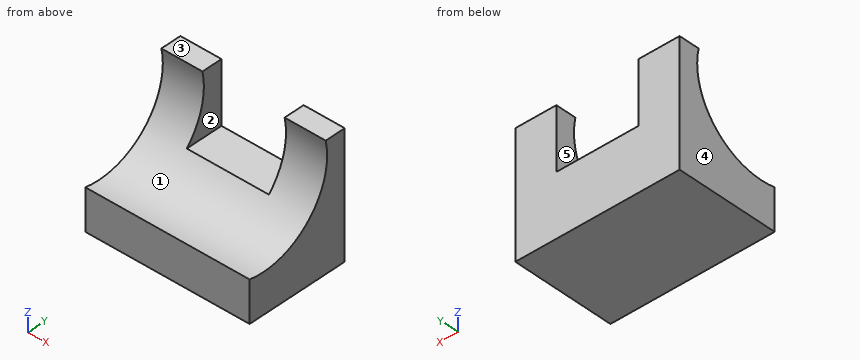
from build123d import *

# Parameters (mm, degrees)
F0_W      = 101.6
F0_H      = 76.2
F1_DEPTH  = 63.5
F3_DEPTH  = 101.6
F4_W      = 50.8
F4_H      = 12.7
F5_DEPTH  = 38.1
F5_FACE_W = 50.8
F5_FACE_H = 20.105892
F6_DEPTH  = 25.4


with BuildPart() as f1:
    # F0 (on Front) → F1 (new body)
    with BuildSketch(Plane.XZ):
        with Locations((-0.270213, -2.291896)):
            Rectangle(F0_W, F0_H)
    extrude(amount=F1_DEPTH)

    # F2 (on face) → F3 (cut)
    with BuildSketch(Plane(origin=(-51.070213, 0, 0), x_dir=(0, -1, 0), z_dir=(-1, 0, 0))):
        with BuildLine():
            Line((63.5, 35.808104), (12.7, 35.808104))
            ThreePointArc((12.7, 35.808104), (24.26693, -3.424965), (63.5, -14.991896))
            Line((63.5, -14.991896), (63.5, 35.808104))
        make_face()
    extrude(amount=-F3_DEPTH, mode=Mode.SUBTRACT)

    # F4 (on face) → F5 (cut)
    with BuildSketch(Plane.XY.offset(35.808104)):
        with Locations((-0.270213, -6.35)):
            Rectangle(F4_W, F4_H)
    extrude(amount=-F5_DEPTH, mode=Mode.SUBTRACT)

    # F5_face (on face) → F6 (cut)
    with BuildSketch(Plane(origin=(-0.270213, -12.7, 7.76105), x_dir=(-1, 0, 0), z_dir=(0, 1, 0))):
        Rectangle(F5_FACE_W, F5_FACE_H)
    extrude(amount=-F6_DEPTH, mode=Mode.SUBTRACT)


solid = f1.part
Source: CAD feature listing. Evaluate the final solid. Frame: model axes, mm. Face numbers are marked on the shaded views. A direction names the side the tool comes from. Coordinates: 2 decimals unless noted, no trailing zeros. Loops run counter-clockwise (first coordinate to the right, second up) from the corner with the lowest first, then second, coordinate; pieces in that order, holes last. Notation, with made-up numbers: (72, 49) - (116, 49) arc R20 ccw to (116, 87) - close; hole circle Ø10 at (30, -5). An arc over 180 degrees is marked (long way). One line per item, written item: value. Start each with the question number.
1. Mould query, pull axis X, two halves, no side actions, for the marked faces 3, 4 and 5. Classes: pulls with the +X half, pulls with the -X half, needs draft (parallel to the pull), parting line crosses it, or undercut.
2. Ray query, L1, parallel to X at y = -6.5, z = 27; L2, parallel to Z at x = 20, y = -7.5; L3, parallel to Z at x = -2.5, y = -36. Return the intervals inside material, ascending.
3. Section C-C (y = -21.5). Return the cut outline in (x, z), and give its area (3 significant figures).
4. Set-up query: the marked faces 1 and 2. Return all of +Z, -Z, +X, -X, +Y, -Y with unobstructed straight access to the full face (end or side cutting, diameter ignored); none if empty.
5. Contact query for flat-ended pins moving along their axis: P1, Ø8, axis at x = -14, z = -7.5, coming from the -Y side; P2, Ø1.5, axis at x = -30.5, y = -37, coming from the +Z side; P3, Ø11.5, axis at x = 3.5, y = -11, coming from the +Z side. Output: stop coordinate, or through.
6. Section A-A (z = 25). Return the cut outline in (x, y), and give its area (3 significant figures).
7. Section D-D (z = 4.5). Return the cut outline in (x, y).
8. Section B-B (x = -22). Return the cut outline in (y, z), and give its area (3 significant figures).
Verdict:
1. face 3: needs draft
1. face 4: pulls with the -X half
1. face 5: undercut
2. L1: x = -51.07 to -25.67, 25.13 to 50.53
2. L2: z = -40.39 to -2.29
2. L3: z = -40.39 to -11.74
3. outline: (-51.07, -40.39) - (50.53, -40.39) - (50.53, -0.38) - (25.13, -0.38) - (25.13, -2.29) - (-25.67, -2.29) - (-25.67, -0.38) - (-51.07, -0.38) - close
3. area: 3,970 mm2
4. face 1: +X, -X
4. face 2: +Z, +Y, -Y
5. P1: stops at y = -35.51
5. P2: stops at z = -11.86
5. P3: stops at z = -2.29
6. outline: (-51.07, -11.78) - (-25.67, -11.78) - (-25.67, 0) - (-51.07, 0) - close; (25.13, -11.78) - (50.53, -11.78) - (50.53, 0) - (25.13, 0) - close
6. area: 598 mm2
7. outline: (-51.07, -18.02) - (-25.67, -18.02) - (-25.67, 0) - (-51.07, 0) - close; (25.13, -18.02) - (50.53, -18.02) - (50.53, 0) - (25.13, 0) - close
8. outline: (-63.5, -40.39) - (0, -40.39) - (0, -2.29) - (-23.17, -2.29) arc R42.76 cw to (-63.5, -14.99) - close
8. area: 2,000 mm2
